The listing builds one solid part. Answer for the finished solid, in the listing's coordinates (mm). A direction names the side the tool comes from. Give positions to 0.01 mm unless a question says otherwise; leave off trailing zeros. Write each loop counter-clockwise with the first axis right and the second up, starting at its lowest first coordinate (ties: lowest second). Pieces come first, ordered by that corner, then holes. Notation, with made-up numbers: (46.5, -33.5) - (88.5, -33.5) arc R31 ccw to (88.5, -9.5) - close; hole circle Ø11 at (79, 18.25). An arc over 180 degrees is marked (long way). Write each question's results on one line, items separated by ' | '. Start each with the question number.
Q1. For faces 1 (the face through (42.4, -1, -6)), 2 (the face through (28, 4, 0)), 3 (the face through (40, -1, -3)), 4 (the face through (27.322, 14.353, -8.646)), determine the directions among +Z, -Z, +X, -X, +Y, -Y from which every point of the face is accessible in a straight line to the end or side of a thin tool.
Q2. Find the intervals of material crossed by probe 1 along Y at (x, z) = (2.4, 0); probe 2 along Z at (x, y) = (40, 3); probe 3 along Y at (x, z) = (6, -9), in increasing order.
Q3. Section D-D (z = 5.75) is taken. Determine the outline of the cut face in (x, y), plus the area to 3 significant figures.
Q4. For a pull along Z with two mould halves and no side action, classify faces 5 (the face through (40, -1, 3)), 6 (the face through (19, 9, -10)), 7 (the face through (42.4, -1, 7)), 8 (the face through (19, 9, 10)) as pulls with the +Z half, pulls with the -Z half, needs draft (parallel to the pull), parting line crosses it, or undercut.
Q5. Section B-B (y = 20) is taken. Determine the outline of the cut face in (x, z).
Q6. Flat-ended cylindrical pins translate along their axes: pin 1 Ø4 at (y, z) = (20, 0) entering from +X; pin 2 Ø4.5 at (y, z) = (10, 0) entering from -X; pin 3 Ø4 at (x, z) = (15, 6) entering from -Y; pin 4 Ø3.5 at (x, z) = (40, 0) entering from +Y. Find the tip coordinate at first contact, or state that the pin passes through.
Q7. Section A-A (z = 0) is taken. Determine the outline of the cut face in (x, y), plus the area to 3 significant figures.
Q8. Section C-C (x = 40) is taken. Determine the outline of the cut face in (y, z), plus the area to 3 significant figures.
```python
from build123d import *

# Parameters (mm, degrees)
SALIENTE_EXTRUIR1_DEPTH = 10
CROQUIS7_W              = 6
CROQUIS7_H              = 1.5
CORTAR_EXTRUIR3_DEPTH   = 51
CROQUIS3_R              = 2.75
CORTAR_EXTRUIR1_DEPTH   = 20
CROQUIS4_R              = 1.8
CORTAR_EXTRUIR2_DEPTH   = 20
SALIENTE_EXTRUIR2_DEPTH = 3
REDONDEO1_R             = 2


with BuildPart() as part:
    # Croquis1 → Saliente-Extruir1 (new body, symmetric)
    with BuildSketch(Plane.XY):
        Polygon((0, 0), (37.4, 0), (38.9, -1.5), (42.4, -1.5), (42.4, 0), (50, 0), (50, 4), (4, 4), (4, 25), (0, 25), align=None)
    extrude(amount=SALIENTE_EXTRUIR1_DEPTH, both=True)

    # Croquis7 → Cortar-Extruir3 (cut, through all)
    with BuildSketch(Plane(origin=(50, 0, 0), x_dir=(0, 0, -1), z_dir=(1, 0, 0))):
        with Locations((0, -0.75)):
            Rectangle(CROQUIS7_W, CROQUIS7_H)
    extrude(amount=-CORTAR_EXTRUIR3_DEPTH, mode=Mode.SUBTRACT)

    # Croquis3 → Cortar-Extruir1 (cut)
    with BuildSketch(Plane.XZ):
        with Locations((40, 0)):
            Circle(CROQUIS3_R)
    extrude(amount=-CORTAR_EXTRUIR1_DEPTH, mode=Mode.SUBTRACT)

    # Croquis4 → Cortar-Extruir2 (cut)
    with BuildSketch(Plane(origin=(4, 0, 0), x_dir=(0, 0, -1), z_dir=(1, 0, 0))):
        with Locations((0, 20)):
            Circle(CROQUIS4_R)
        with Locations((0, 10)):
            Circle(CROQUIS4_R)
    extrude(amount=-CORTAR_EXTRUIR2_DEPTH, mode=Mode.SUBTRACT)

    # Croquis5 → Saliente-Extruir2 (add)
    with BuildSketch(Plane(origin=(0, 0, -10), x_dir=(-1, 0, 0), z_dir=(0, 0, -1))):
        Polygon((0, 0), (-50, 0), (-50, 4), (-4, 25), (0, 25), align=None)
    saliente_extruir2 = extrude(amount=-SALIENTE_EXTRUIR2_DEPTH)

    # Simetría1: Saliente-Extruir2 across plane
    add(saliente_extruir2.mirror(Plane.XY))

    # Redondeo1
    redondeo1_edges = [part.edges().sort_by_distance(p)[0] for p in [
        (4, 14.5, 7),
        (27, 4, 7),
        (27, 4, -7),
        (4, 14.5, -7),
        (4, 4, 0),
    ]]
    fillet(redondeo1_edges, radius=REDONDEO1_R)


solid = part.part
```
Answers below:
1) face 1: +Z, -Z, +X, -Y | face 2: +X, +Y | face 3: +X, -X, -Y | face 4: +Z, -Z, +X, +Y
2) probe 1: y = 0 to 8.2, 11.8 to 18.2, 21.8 to 25 | probe 2: z = -10 to -2.75, 2.75 to 10 | probe 3: y = 0 to 24.09
3) outline: (0, 0) - (37.4, 0) - (38.9, -1.5) - (42.4, -1.5) - (42.4, 0) - (50, 0) - (50, 4) - (49.68, 4.15) - (6, 4.15) arc R1.85 cw to (4.15, 6) - (4.15, 24.93) - (4, 25) - (0, 25) - close | area: 301 mm2
4) face 5: undercut | face 6: pulls with the -Z half | face 7: needs draft | face 8: pulls with the +Z half
5) outline: (0, -10) - (14.95, -10) - (14.95, -7) - (6, -7) arc R2 cw to (4, -5) - (4, -1.8) - (0, -1.8) - close; (0, 1.8) - (4, 1.8) - (4, 5) arc R2 cw to (6, 7) - (14.95, 7) - (14.95, 10) - (0, 10) - close
6) pin 1: stops at x = 4 | pin 2: stops at x = 0 | pin 3: stops at y = 0 | pin 4: passes through
7) outline: (0, 0) - (37.25, 0) - (37.25, 4) - (6, 4) arc R2 cw to (4, 6) - (4, 8.2) - (0, 8.2) - close; (0, 11.8) - (4, 11.8) - (4, 18.2) - (0, 18.2) - close; (0, 21.8) - (4, 21.8) - (4, 25) - (0, 25) - close; (42.75, 0) - (50, 0) - (50, 4) - (42.75, 4) - close | area: 234 mm2
8) outline: (-1.5, -10) - (8.57, -10) - (8.57, -7) - (6, -7) arc R2 cw to (4, -5) - (4, -2.75) - (0, -2.75) - (0, -3) - (-1.5, -3) - close; (-1.5, 3) - (0, 3) - (0, 2.75) - (4, 2.75) - (4, 5) arc R2 cw to (6, 7) - (8.57, 7) - (8.57, 10) - (-1.5, 10) - close | area: 108 mm2
